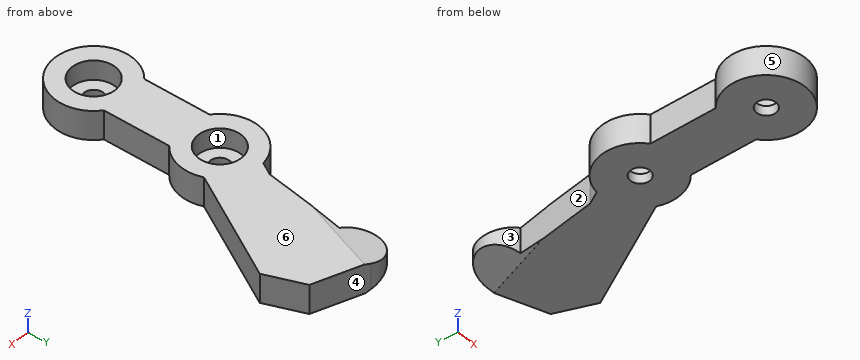
```python
from build123d import *

# Parameters (mm, degrees)
BOSS_EXTRUDE1_DEPTH     = 15
SKETCH2_R               = 11.1
CUT_EXTRUDE1_DEPTH      = 10
SKETCH3_R               = 5
CUT_EXTRUDE2_DEPTH      = 10
CUT_EXTRUDE_THIN3_DEPTH = 63


with BuildPart() as part:
    # Sketch1 → Boss-Extrude1 (new body)
    with BuildSketch(Plane.XY):
        with BuildLine():
            Line((5.505816945, 85.326012217), (5.307768654, 85.393580353))
            ThreePointArc((5.307768654, 85.393580353), (-2.005055015, 101.475976607), (13.940536847, 109.082484312))
            Line((13.940536847, 109.082484312), (40.538740524, 99.7887516))
            Line((40.538740524, 99.7887516), (48.129208704, 80.495248668))
            Line((48.129208704, 80.495248668), (17.636215156, 25.115965593))
            ThreePointArc((17.636215156, 25.115965593), (18.579608232, 12.6739017), (11.964278199, 2.09409296))
            Line((11.964278199, 2.09409296), (12.243619866, -31.678974911))
            ThreePointArc((12.243619866, -31.678974911), (0.468324559, -67.537617109), (-12.751239862, -32.185913949))
            Line((-12.751239862, -32.185913949), (-13.03091257, 1.603476045))
            ThreePointArc((-13.03091257, 1.603476045), (-20.259022529, 22.242640416), (-4.270337109, 37.161843413))
            Line((-4.270337109, 37.161843413), (-0.71558036, 43.617748767))
            Line((-0.71558036, 43.617748767), (5.505816945, 85.326012217))
        make_face()
    extrude(amount=BOSS_EXTRUDE1_DEPTH)

    # Sketch2 → Cut-Extrude1 (cut)
    with BuildSketch(Plane.XY.offset(15)):
        with Locations((-0.839707244, 17.458270673)):
            Circle(SKETCH2_R)
        with Locations((0.062773329, -47.541729327)):
            Circle(SKETCH2_R)
    extrude(amount=-CUT_EXTRUDE1_DEPTH, mode=Mode.SUBTRACT)

    # Sketch3 → Cut-Extrude2 (cut)
    with BuildSketch(Plane.XY.offset(5)):
        with Locations((-0.839707244, 17.458270673)):
            Circle(SKETCH3_R)
        with Locations((0.062773329, -47.541729327)):
            Circle(SKETCH3_R)
    extrude(amount=-CUT_EXTRUDE2_DEPTH, mode=Mode.SUBTRACT)

    # Sketch6 → Cut-Extrude-Thin3 (cut)
    with BuildSketch(Plane(origin=(35.484462303, 101.554777284, 0), x_dir=(0.944031293, -0.329855904, 0), z_dir=(0.329855904, 0.944031293, 0))):
        Polygon((-20.418832703, -0.085187968), (-37.64557492, -6.976961591), (-41.359981954, 2.307605194), (-24.133239737, 9.199378817), align=None)
        Polygon((-37.640333131, -10.87506916), (-19.777391753, -14.888150458), (-21.969352424, -24.644958769), (-39.832293801, -20.631877471), align=None)
    extrude(amount=-CUT_EXTRUDE_THIN3_DEPTH, mode=Mode.SUBTRACT)


solid = part.part
```
Geometry check sheet. Reference: the model listing, model coordinates, mm. Face numbers are marked on the shaded views. A direction names the side the tool comes from. Round coordinates to 2 decimals unless told otherwise and drop trailing zeros. Loops run counter-clockwise (first coordinate to the right, second up) from the corner with the lowest first, then second, coordinate; pieces in that order, holes last. Notation, with made-up numbers: M 29,32.5 L 66,32.5 A16 cw 66,58.5 Z; hole C 58.25,82 d6. An arc over 180 degrees is marked long. Return JSON: item names as keys, results as strings. Group by question number.
(1) Section check C-C, the plane x = 7.5. Enter the section's corners in (y, z), and give its area (3 significant figures).
(2) Section check B-B, the plane y = 77. Enter the section's corners in (x, z), and give its area (3 significant figures).
(3) Section check A-A, the plane z = 8.5. Enter the section's corners in (x, y).
(4) Mould release check, pull along Y, two halves, no side actions. Record for the marked faces 4, 5 and 6: pulls with the +Y half, pulls with the -Y half, needs draft (parallel to the pull), parting line crosses it, or undercut.
(5) Go/stop test with flat-tipped pins: pin 1 (9 mm diameter, centred on x = 0.06, y = -47.54, fed in from -Z); pin 2 (2 mm diameter, centred on y = 50, z = 8.5, fed in from -X); pin 3 (2 mm diameter, centred on y = 4.5, z = 11, fed in from -X); pin 4 (1 mm diameter, centred on y = 44, z = 3, fed in from +X). Record where each tip stops, or that it passes through.
(6) Section check D-D, the plane x = 43. Enter the section's corners in (y, z), and give its area (3 significant figures).
(7) Set-up check for the marked faces 1, 2 and 3: record each of +Z, -Z, +X, -X, +Y, -Y from which the full face is reachable in a straight line by a thin tool's end or side.
(8) Scan lines: line 1 along Y through (x, z) = (-2, 13.75); line 2 along Z through (x, y) = (8.5, -43); line 3 along Y through (x, z) = (-15, 8.25). Record each from-to range of solid material in increasing order. Write a range as [from, to].
Data:
{
 "1": {"outline": "M -66.11,0 L 83.47,0 L 83.37,0.09 L 109.55,3.54 L 109.55,12.8 L 81.42,14.89 L 81.5,15 L 24.78,15 L 24.78,5 L 10.13,5 L 10.13,15 L -39.3,15 L -39.3,5 L -55.78,5 L -55.78,15 L -66.11,15 Z", "area": "2,240 mm²"},
 "2": {"outline": "M 4.26,0.47 L 5.28,0.09 L 5.24,0 L 46.2,0 L 46.2,15 L 5.93,15 L 5.95,14.89 L 4.26,14.53 Z", "area": "628 mm²"},
 "3": {"outline": "M -13.03,1.6 L -12.75,-32.19 A20 ccw long 12.24,-31.68 L 11.96,2.09 A20 ccw 17.64,25.12 L 48.13,80.5 L 40.54,99.79 L 13.94,109.08 A12.61 ccw 5.31,85.39 L 5.51,85.33 L -0.72,43.62 L -4.27,37.16 A20 ccw Z; hole C -0.84,17.46 d22.2; hole C 0.06,-47.54 d22.2"},
 "4": {"face 4": "pulls with the +Y half", "face 5": "undercut", "face 6": "needs draft"},
 "5": {"pin 1": "through", "pin 2": "x = 0.09", "pin 3": "x = -16.87", "pin 4": "x = 28.31"},
 "6": {"outline": "M 71.18,0 L 93.53,0 L 93.53,15 L 71.18,15 Z", "area": "335 mm²"},
 "7": {"face 1": "+Z", "face 2": "+Z, -Z, -X", "face 3": "+Z, -Z"},
 "8": {"line 1": "[-67.44, -58.45], [-36.64, 6.42], [28.5, 41.29]", "line 2": "[0, 5]", "line 3": "[-60.7, -34.38], [3.33, 31.58]"}
}
